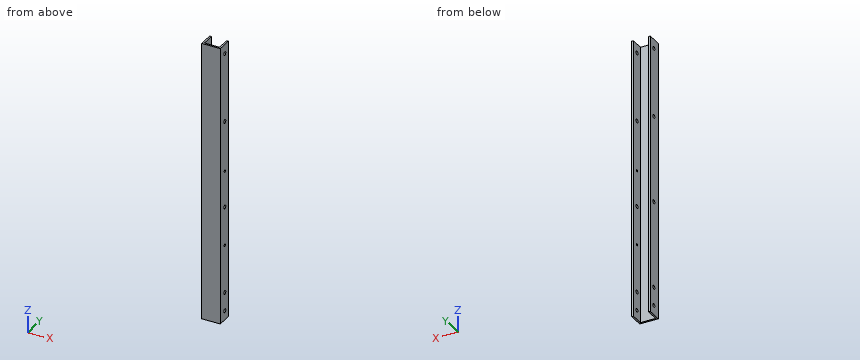
Autodesk Inventor part; units mm, degrees
ref_plane "YZ Plane" through (0, 0, 0) normal (1, 0, 0) x (0, 1, 0)
ref_plane "XZ Plane" through (0, 0, 0) normal (0, 1, 0) x (-1, 0, 0)
ref_plane "XY Plane" through (0, 0, 0) normal (0, 0, 1) x (1, 0, 0)
sketch "Sketch1" plane through (0, 0, 0) normal (0, 0, 1) x (1, 0, 0)
  line L0 (-16, 12.5) -> (-13, 12.5)
  line L1 (-13, 12.5) -> (-13, -9.5)
  line L2 (-13, -9.5) -> (13, -9.5)
  line L3 (13, -9.5) -> (13, 12.5)
  line L4 (13, 12.5) -> (16, 12.5)
  line L5 (16, 12.5) -> (16, -12.5)
  line L6 (16, -12.5) -> (-16, -12.5)
  line L7 (-16, -12.5) -> (-16, 12.5)
  point P0 (0, 0)
  dimension "d0" = 3
  dimension "d2" = 3
  dimension "d3" = 25
  dimension "d4" = 32
  dimension "d5" = 16
  dimension "d7" = 12.5
  dimension "d8" = 3
  dimension "d53" = 25
extrude "Extrusion1" add sketch "Sketch1" against normal blind 482.6
sketch "Sketch12" plane through (16, -12.5, 0) normal (1, 0, 0) x (0, 0, -1)
  circle A0 centre (16, 14) radius 3.175
  circle A1 centre (16, 14) radius 3.175
  circle A2 centre (466.6, 14) radius 3.175
  circle A3 centre (466.6, 14) radius 3.175
  circle A4 centre (135, 14) radius 3.175
  circle A5 centre (135, 14) radius 3.175
  circle A6 centre (434.6, 14) radius 3.175
  circle A7 centre (284.8, 14) radius 3.175
  point P0 (0, 12.5)
hole "Hole2" at (16, 1.5, -16) at (16, 1.5, -466.6) at (16, 1.5, -135) at (16, 1.5, -434.6) at (16, 1.5, -284.8) direction (-1, 0, 0) diameter 6.35 end through all
sketch "Sketch13" plane through (16, -12.5, 0) normal (1, 0, 0) x (0, 0, -1)
  circle A0 centre (351.875, 14.0056) radius 2
  circle A1 centre (221.9249, 14.017) radius 2
  point P0 (0, 12.5)
hole "Hole3" at (16, 1.5056, -351.875) at (16, 1.517, -221.9249) direction (-1, 0, 0) diameter 4 depth 3 tip angle 118
equation "\"d2\" = d0"
equation "\"d8\" = d0"
equation "\"d53\" = d3"
properties part number "18in C-Channel Front" material "Aluminum 6061"
Read the model definition and answer for the solid it produces. Units are mm, in the model's axes. Round coordinates to 2 decimals unless told otherwise and drop trailing zeros. Write each loop counter-clockwise with the first axis right and the second up, starting at its lowest first coordinate (ties: lowest second). Pieces come first, ordered by that corner, then holes. Notation, with made-up numbers: (39, 12.5) - (53, 12.5) arc R19 ccw to (53, 18.5) - close; hole circle Ø3 at (24, 0.25). An arc over 180 degrees is marked (long way). One line per item, written item: value.
Q1. Each of these flat-tipped pins is pushed along its axis until it touches: P1, Ø7.5, axis at y = 1.5, z = -466.6, coming from the -X side; P2, Ø6, axis at x = 1, z = -411, coming from the +Y side; P3, Ø2.5, axis at y = 1.51, z = -351.88, coming from the +X side. Where does it stop, or does it pass through?
The answers:
P1: stops at x = -16
P2: stops at y = -9.5
P3: stops at x = -13
Q2. Find section A-A (z = -310.5). Determine the outline of the cut face in (x, y), and give its area (3 significant figures).
The answers:
outline: (-16, -12.5) - (16, -12.5) - (16, 12.5) - (13, 12.5) - (13, -9.5) - (-13, -9.5) - (-13, 12.5) - (-16, 12.5) - close
area: 228 mm2
Q3. Straight lines are drawn through the part: line 1 (Z direction, x = -15.2, y = 1.5) (3 decimals); line 2 (Y direction, x = -15, z = -466); line 3 (Y direction, x = -15.3, z = -16) (3 decimals). For each, find the intervals that lie inside material, in ascending order. Write a range as from..to.
The answers:
line 1: z = -482.6..-469.775, -463.425..-437.775, -431.425..-287.975, -281.625..-138.175, -131.825..-19.175, -12.825..0
line 2: y = -12.5..-1.62, 4.62..12.5
line 3: y = -12.5..-1.675, 4.675..12.5
Q4. Find section B-B (x = -1). Determine the outline of the cut face in (y, z).
The answers:
outline: (-12.5, -482.6) - (-9.5, -482.6) - (-9.5, 0) - (-12.5, 0) - close
